Read the model definition and answer for the solid it produces. Units are mm, in the model's axes. A direction names the side the tool comes from. Give positions to 0.01 mm unless a question says otherwise; leave off trailing zeros. Write each loop counter-clockwise with the first axis right and the second up, starting at its lowest first coordinate (ties: lowest second). Pieces come first, ordered by that corner, then holes. Notation, with made-up numbers: M -10,76.25 L -5,76.25 A21 ccw -5,106.25 Z; hole C 58,60.25 d1. An arc over 180 degrees is marked long. Use a Markdown table: item, result. Add a question column.
Item 1: Given P1, Ø4, axis at x = -20, y = -56.5, coming from the -Z side; P2, Ø6, axis at y = -53, z = -68, coming from the +X side; P3, Ø3, axis at x = 0.5, z = -68, coming from the -Y side; P4, Ø1.9, axis at y = -59.5, z = -74.5, coming from the +X side, each flat-ended and moving along its own axis, determine where each tip first touches the part or whether it passes through.
Item 2: The mould has two halves that part along Y. Classify faces 1 (the cylindrical face through (-49.244, -55.839, -69.347)), 2 (the flat face through (35.21, -53.3, -65.6)), 3 (the cylindrical face through (-54.45, -58.32, -72.89)): pulls with the +Y half, pulls with the -Y half, needs draft (parallel to the pull), parting line crosses it, or undercut.
Item 3: For faces 4 (the flat face through (-0.6, -58.7, -73.4)), 5 (the flat face through (-0.479, -53.864, -66.405)), 6 (the cylindrical face through (54.353, -58.375, -72.968)), determine the directions among +Z, -Z, +X, -X, +Y, -Y from which every point of the face is accessible in a straight line to the end or side of a thin tool.
Item 4: Consider probe 1 along X at (y, z) = (-54.5, -69); probe 2 along X at (y, z) = (-57.75, -70.25); probe 3 along X at (y, z) = (-57.75, -75). Determine where each line is inside the solid, lowest interval first. Write a range as [from, to].
Item 5: A cutting plane is placed at B-B on x = 48. Determine the outline of the cut face in (y, z), then the cut area to 3 significant figures.
Item 6: A cutting plane is placed at A-A on x = 25. Determine the outline of the cut face in (y, z).
from build123d import *

# Parameters (mm, degrees)
SKETCH1_R             = 2
BOSS_EXTRUDE1_DEPTH   = 5
BOSS_EXTRUDE1_2_DEPTH = 5
SKETCH2_W             = 72.454585158
SKETCH2_H             = 8.503113073
BOSS_EXTRUDE2_DEPTH   = 5
CHAMFER1_SIZE         = 2
FILLET1_R             = 6


# Some blends are built 0.0001 mm under size
with BuildPart() as part:
    # Sketch1 → Boss-Extrude1 (new body)
    with BuildSketch(Plane(origin=(0, -2.867032155, 2.007517527), x_dir=(1, 0, 0), z_dir=(0, -0.8191520442889961, 0.5735764363510402))):
        Polygon((-56.227292579, -83.290902945), (-56.227292579, -94.897888962), (-46.227292579, -94.897888962), (-46.227292579, -93.794016018), (-36.227292579, -93.794016018), (-36.227292579, -83.290902945), align=None)
        with Locations(Location((-51.227292579, -89.094395953, 0), (0, 0, 270))):
            Circle(SKETCH1_R, mode=Mode.SUBTRACT)
    extrude(amount=BOSS_EXTRUDE1_DEPTH)



with BuildPart() as body_2:
    # Sketch1 → Boss-Extrude1 2 (new body)
    with BuildSketch(Plane(origin=(0, -2.867032155, 2.007517527), x_dir=(1, 0, 0), z_dir=(0, -0.8191520442889961, 0.5735764363510402))):
        Polygon((36.227292579, -83.290902945), (56.227292579, -83.290902945), (56.227292579, -94.897888962), (46.227292579, -94.897888962), (46.227292579, -93.794016018), (36.227292579, -93.794016018), align=None)
        with Locations(Location((51.227292579, -89.094395953, 0), (0, 0, 90))):
            Circle(SKETCH1_R, mode=Mode.SUBTRACT)
    extrude(amount=BOSS_EXTRUDE1_2_DEPTH)


with BuildPart() as part_1:
    add(part.part)

    add(body_2.part)  # Boss-Extrude2 merges body 2
    # Sketch2 → Boss-Extrude2 (add)
    with BuildSketch(Plane(origin=(0, -6.962792376, 4.875399709), x_dir=(1, 0, 0), z_dir=(0, -0.8191520442889959, 0.5735764363510404))):
        with Locations((0, -89.542459482)):
            Rectangle(SKETCH2_W, SKETCH2_H)
    extrude(amount=-BOSS_EXTRUDE2_DEPTH)

    # Chamfer1
    chamfer1_edges = [part_1.edges().sort_by_distance(p)[0] for p in [
        (36.227292579, -53.83576443, -66.424758888),
        (-36.227292579, -53.83576443, -66.424758888),
    ]]
    chamfer(chamfer1_edges, length=CHAMFER1_SIZE - 0.0001)  # a hair under: the kernel refuses the full size

    # Fillet1
    # the kernel refuses this fillet: 6 mm, written as the material it takes off along each edge
    with BuildSketch(Plane(origin=(56.227292579, -45.010944459, -84.33192876), x_dir=(1.184237892933516e-15, 0.5735764363510399, 0.819152044288996), z_dir=(0, -0.819152044288996, 0.57357643635104)), Plane(origin=(56.227292579, -38.353450782, -74.824042436), x_dir=(-1, 0, 0), z_dir=(0, -0.819152044288996, 0.57357643635104))) as fillet1_piece_1:
        with BuildLine():
            CenterArc((FILLET1_R, FILLET1_R), FILLET1_R, 180, 90)
            Line((0, FILLET1_R), (0, 0))
            Line((0, 0), (FILLET1_R, 0))
        make_face()
    extrude(amount=35, mode=Mode.SUBTRACT)
    with BuildSketch(Plane(origin=(-56.227292579, -38.353450782, -74.824042436), x_dir=(1, 0, 0), z_dir=(0, -0.819152044288996, 0.57357643635104)), Plane(origin=(-56.227292579, -45.010944459, -84.33192876), x_dir=(0, 0.57357643635104, 0.819152044288996), z_dir=(0, -0.819152044288996, 0.57357643635104))) as fillet1_piece_2:
        with BuildLine():
            CenterArc((FILLET1_R, -FILLET1_R), FILLET1_R, 90, 90)
            Line((0, -FILLET1_R), (0, 0))
            Line((0, 0), (FILLET1_R, 0))
        make_face()
    extrude(amount=35, mode=Mode.SUBTRACT)


solid = part_1.part
Filled in:
| question | item | result |
|---|---|---|
| 1 | P1 | z = -74.82 |
| 1 | P2 | x = 56.22 |
| 1 | P3 | y = -59.04 |
| 1 | P4 | x = 53.03 |
| 2 | face 1 | undercut |
| 2 | face 2 | pulls with the +Y half |
| 2 | face 3 | pulls with the -Y half |
| 3 | face 4 | -Z, -Y |
| 3 | face 5 | +Z, +Y |
| 3 | face 6 | -Z, +X, -Y |
| 4 | probe 1 | [-56.03, -52.74], [-49.72, 49.72], [52.74, 56.03] |
| 4 | probe 2 | [-55.96, -52.46], [-49.99, 49.99], [52.46, 55.96] |
| 4 | probe 3 | [-52.21, -46.23], [46.23, 52.21] |
| 5 | outline | M -61.39,-72.86 L -57.3,-75.73 L -50.64,-66.22 L -54.74,-63.35 Z |
| 5 | area | 58.0 mm² |
| 6 | outline | M -60.76,-71.96 L -56.67,-74.82 L -51.79,-67.86 L -55.88,-64.99 Z |
